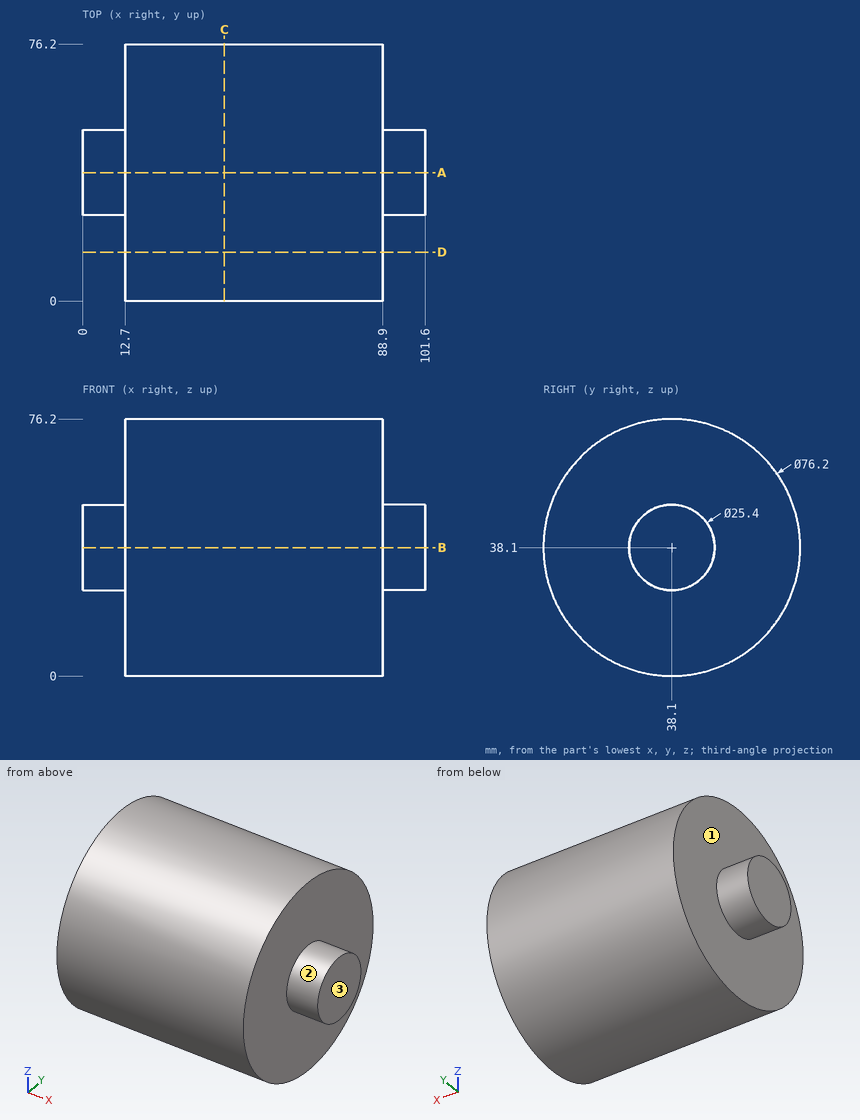
Check sheet for the drawn part. Datum: minimum x, y, z corner. Units: mm. A direction names the side the tool comes from. Give positions to 0.01 mm unless a question says otherwise; leave off trailing zeros. Write each loop counter-clockwise with the first axis right and the second up, starting at its lowest first coordinate (ties: lowest second). Pieces come first, ordered by that corner, then holes. Notation, with made-up numbers: M 2,36 L 57,36 A24 cw 57,58 Z; hole C 47,-6 d6. An arc over 180 degrees is marked long. One line per question, with ' | ' between items.
1) Section check A-A on y = 38.1. Enter the section's corners in (x, z).
Result:
outline: M 0,25.4 L 12.7,25.4 L 12.7,0 L 88.9,0 L 88.9,25.4 L 101.6,25.4 L 101.6,50.8 L 88.9,50.8 L 88.9,76.2 L 12.7,76.2 L 12.7,50.8 L 0,50.8 Z
2) Section check C-C on x = 42. Enter the section's corners in (y, z).
Result:
outline: C 38.1,38.1 d76.2
3) Set-up check for the marked faces 1, 2 and 3: record each of +Z, -Z, +X, -X, +Y, -Y from which the full face is reachable in a straight line by a thin tool's end or side.
Result:
face 1: -X | face 2: +X | face 3: +Z, -Z, +X, +Y, -Y
4) Section check D-D on y = 14.5. Enter the section's corners in (x, z), plus the area to 3 significant figures.
Result:
outline: M 12.7,8.19 L 88.9,8.19 L 88.9,68.01 L 12.7,68.01 Z | area: 4,560 mm2
5) Gauge pin test, flat ends, axial feed: pin 1 Ø1.5 at (x, y) = (74, 33) entering from +Z; pin 2 Ø2 at (x, y) = (69, 67.5) entering from -Z; pin 3 Ø2 at (x, z) = (80.5, 23) entering from +Y. Record the tip position at first contact, or that the pin passes through.
Result:
pin 1: stops at z = 75.95 | pin 2: stops at z = 12.7 | pin 3: stops at y = 73.49
6) Thickness scan on line 1 along X through (y, z) = (16, 11.5); line 2 along Z through (x, y) = (34.5, 56); line 3 along Z through (x, y) = (56.5, 22.5). Record the ranges inside material, lowest first. Write a range as [from, to].
Result:
line 1: x = [12.7, 88.9] | line 2: z = [4.47, 71.73] | line 3: z = [3.34, 72.86]
